Work out the finished part from the listing and answer in its coordinate system (mm). Coordinates: 2 decimals unless noted, no trailing zeros. Loops run counter-clockwise (first coordinate to the right, second up) from the corner with the lowest first, then second, coordinate; pieces in that order, holes last. Notation, with made-up numbers: (-11.5, 82) -> (19.5, 82) arc R18 cw to (19.5, 103) -> close; hole circle Ø7 at (-6, 55.25). An arc over 180 degrees is marked (long way). Use a Markdown table: item, result.
from build123d import *

# Parameters (mm, degrees)
BOSS_EXTRUDE1_DEPTH = 19.08


with BuildPart() as part:
    # Sketch15 → Boss-Extrude1 (new body)
    with BuildSketch(Plane(origin=(0, 0, 0), x_dir=(1, 0, 0), z_dir=(0, 1, 0))):
        with BuildLine():
            Line((0, 9.54), (1200, 9.54))
            ThreePointArc((1200, 9.54), (1209.050438663, 3.016812888), (1205.724, -7.632))
            Line((1205.724, -7.632), (805.724, -307.632))
            ThreePointArc((805.724, -307.632), (803.016812888, -309.050438663), (800, -309.54))
            Line((800, -309.54), (400, -309.54))
            ThreePointArc((400, -309.54), (396.983187112, -309.050438663), (394.276, -307.632))
            Line((394.276, -307.632), (-5.724, -7.632))
            ThreePointArc((-5.724, -7.632), (-9.050438663, 3.016812888), (0, 9.54))
        make_face()
        Polygon((390.46, -280.92), (390.46, -9.54), (28.62, -9.54), align=None, mode=Mode.SUBTRACT)
        Polygon((409.54, -19.08), (409.54, -290.46), (771.38, -290.46), align=None, mode=Mode.SUBTRACT)
        Polygon((790.46, -280.921851045), (428.61753194, -9.54), (790.46, -9.54), align=None, mode=Mode.SUBTRACT)
        Polygon((809.54, -280.92), (1171.38, -9.54), (809.54, -9.54), align=None, mode=Mode.SUBTRACT)
    extrude(amount=BOSS_EXTRUDE1_DEPTH)


solid = part.part
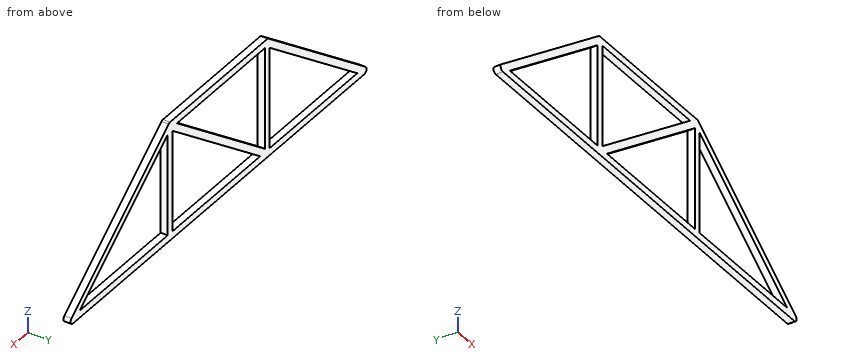
Q1. Section A-A on y = 5.75 is taken. Determine the outline of the cut face in (x, z).
Solved:
| item | result |
|---|---|
| outline | (-5.72, 7.63) arc R9.54 ccw to (0, -9.54) -> (1200, -9.54) arc R9.54 ccw to (1205.72, 7.63) -> (805.72, 307.63) arc R9.54 ccw to (800, 309.54) -> (400, 309.54) arc R9.54 ccw to (394.28, 307.63) -> close; hole (28.62, 9.54) -> (390.46, 9.54) -> (390.46, 280.92) -> close; hole (409.54, 19.08) -> (771.38, 290.46) -> (409.54, 290.46) -> close; hole (428.62, 9.54) -> (790.46, 9.54) -> (790.46, 280.92) -> close; hole (809.54, 9.54) -> (1171.38, 9.54) -> (809.54, 280.92) -> close |
Q2. Consider line 1 (Z direction, x = 739, y = 17.5) (3 decimals); line 2 (X direction, y = 5.5, z = 47); line 3 (X direction, y = 7.25, z = 196). Determine where each line is inside the solid, lowest interval first. Write a range as [from, to].
Solved:
| item | result |
|---|---|
| line 1 | [-9.54, 9.54], [242.327, 266.175], [290.46, 309.54] |
| line 2 | [46.77, 78.57], [390.46, 409.54], [446.77, 478.56], [790.46, 809.54], [1121.43, 1153.23] |
| line 3 | [245.43, 277.23], [390.46, 409.54], [645.43, 677.23], [790.46, 809.54], [922.77, 954.57] |
Q3. Section B-B on z = 121.5 is taken. Determine the outline of the cut face in (x, y).
Solved:
| item | result |
|---|---|
| outline | (146.1, 0) -> (177.9, 0) -> (177.9, 19.08) -> (146.1, 19.08) -> close; (390.46, 0) -> (409.54, 0) -> (409.54, 19.08) -> (390.46, 19.08) -> close; (546.1, 0) -> (577.9, 0) -> (577.9, 19.08) -> (546.1, 19.08) -> close; (790.46, 0) -> (809.54, 0) -> (809.54, 19.08) -> (790.46, 19.08) -> close; (1022.1, 0) -> (1053.9, 0) -> (1053.9, 19.08) -> (1022.1, 19.08) -> close |
Q4. Section D-D on x = 521 is taken. Determine the outline of the cut face in (y, z) (3 decimals).
Solved:
| item | result |
|---|---|
| outline | (0, -9.54) -> (19.08, -9.54) -> (19.08, 9.54) -> (0, 9.54) -> close; (0, 78.827) -> (19.08, 78.827) -> (19.08, 102.675) -> (0, 102.675) -> close; (0, 290.46) -> (19.08, 290.46) -> (19.08, 309.54) -> (0, 309.54) -> close |
Q5. Given pin 1 Ø5.5 at (y, z) = (10.5, 172) entering from +X; pin 2 Ø9.5 at (y, z) = (8.5, 85.5) entering from -X; pin 3 Ø5.5 at (y, z) = (6.5, 197) entering from +X, each flat-ended and moving along its own axis, determine where each tip first touches the part or whether it passes through.
Solved:
| item | result |
|---|---|
| pin 1 | x = 990.23 |
| pin 2 | x = 91.77 |
| pin 3 | x = 956.9 |
Q6. Section C-C on x = 115 is taken. Determine the outline of the cut face in (y, z) (3 decimals).
Solved:
| item | result |
|---|---|
| outline | (0, -9.54) -> (19.08, -9.54) -> (19.08, 9.54) -> (0, 9.54) -> close; (0, 74.325) -> (19.08, 74.325) -> (19.08, 98.175) -> (0, 98.175) -> close |
